```python
from build123d import *

# Parameters (mm, degrees)
SALIENTE_EXTRUIR1_DEPTH = 5
CROQUIS2_R              = 1.563071694
CORTAR_EXTRUIR1_DEPTH   = 10


with BuildPart() as part:
    # Croquis1 → Saliente-Extruir1 (new body)
    with BuildSketch(Plane.XY):
        with BuildLine():
            ThreePointArc((-51.415727165, 73.433311131), (-42.744189857, 73.869405728), (-37.96791411, 81.120124849))
            Line((-37.96791411, 81.120124849), (-37.96791411, 86.394261487))
            Line((-37.96791411, 86.394261487), (-19.296868546, 86.394261487))
            Line((-19.296868546, 86.394261487), (-19.296868546, 91.89912361))
            ThreePointArc((-19.296868546, 91.89912361), (-17.466810584, 93.728616325), (-14.967256479, 94.398231899))
            Line((-14.967256479, 94.398231899), (14.931670067, 94.398231899))
            ThreePointArc((14.931670067, 94.398231899), (17.431224172, 93.728616325), (19.261282134, 91.89912361))
            Line((19.261282134, 91.89912361), (19.261282134, 86.402202311))
            Line((19.261282134, 86.402202311), (49.864249238, 86.408504811))
            Line((49.864249238, 86.408504811), (65.171190916, 59.908709118))
            Line((65.171190916, 59.908709118), (69.938541359, 62.661140179))
            ThreePointArc((69.938541359, 62.661140179), (72.437957507, 61.991009851), (74.267638657, 60.161140285))
            Line((74.267638657, 60.161140285), (89.21710193, 34.267910351))
            ThreePointArc((89.21710193, 34.267910351), (89.886974885, 31.768425211), (89.217616699, 29.268802168))
            Line((89.217616699, 29.268802168), (84.457143211, 26.520341518))
            Line((84.457143211, 26.520341518), (99.764084889, 0.020545825))
            Line((99.764084889, 0.020545825), (84.468059462, -26.485552369))
            Line((84.468059462, -26.485552369), (89.235409905, -29.237983431))
            ThreePointArc((89.235409905, -29.237983431), (89.904768091, -31.737606474), (89.234895136, -34.237091613))
            Line((89.234895136, -34.237091613), (74.285431863, -60.130321548))
            ThreePointArc((74.285431863, -60.130321548), (72.455750713, -61.960191114), (69.956334565, -62.630321442))
            Line((69.956334565, -62.630321442), (65.195861077, -59.881860793))
            Line((65.195861077, -59.881860793), (56.094468632, -75.653435114))
            ThreePointArc((56.094468632, -75.653435114), (42.096374739, -72.88292625), (37.495566471, -86.390513573))
            Line((37.495566471, -86.390513573), (19.296868546, -86.394261487))
            Line((19.296868546, -86.394261487), (19.296868546, -91.89912361))
            ThreePointArc((19.296868546, -91.89912361), (17.466810584, -93.728616325), (14.967256479, -94.398231899))
            Line((14.967256479, -94.398231899), (-14.931670067, -94.398231899))
            ThreePointArc((-14.931670067, -94.398231899), (-17.431224172, -93.728616325), (-19.261282134, -91.89912361))
            Line((-19.261282134, -91.89912361), (-19.261282134, -86.402202311))
            Line((-19.261282134, -86.402202311), (-49.864249238, -86.408504811))
            Line((-49.864249238, -86.408504811), (-65.171190916, -59.908709118))
            Line((-65.171190916, -59.908709118), (-69.938541359, -62.661140179))
            ThreePointArc((-69.938541359, -62.661140179), (-72.437957507, -61.991009851), (-74.267638657, -60.161140285))
            Line((-74.267638657, -60.161140285), (-89.21710193, -34.267910351))
            ThreePointArc((-89.21710193, -34.267910351), (-89.886974885, -31.768425211), (-89.217616699, -29.268802168))
            Line((-89.217616699, -29.268802168), (-84.457143211, -26.520341518))
            Line((-84.457143211, -26.520341518), (-99.764084889, -0.020545825))
            Line((-99.764084889, -0.020545825), (-84.468059462, 26.485552369))
            Line((-84.468059462, 26.485552369), (-89.235409905, 29.237983431))
            ThreePointArc((-89.235409905, 29.237983431), (-89.904768091, 31.737606474), (-89.234895136, 34.237091613))
            Line((-89.234895136, 34.237091613), (-74.285431863, 60.130321548))
            ThreePointArc((-74.285431863, 60.130321548), (-72.455750713, 61.960191114), (-69.956334565, 62.630321442))
            Line((-69.956334565, 62.630321442), (-65.195861077, 59.881860793))
            Line((-65.195861077, 59.881860793), (-55.88668677, 76.013702989))
            Line((-55.88668677, 76.013702989), (-51.415727165, 73.433311131))
        make_face()
    extrude(amount=SALIENTE_EXTRUIR1_DEPTH)

    # Croquis2 → Cortar-Extruir1 (cut)
    with BuildSketch(Plane.XY.offset(5)):
        with Locations((40.934728827, -68.058233997)):
            Circle(CROQUIS2_R)
    extrude(amount=-CORTAR_EXTRUIR1_DEPTH, mode=Mode.SUBTRACT)


solid = part.part
```
The listing builds one solid part. Answer for the finished solid, in the listing's coordinates (mm). A direction names the side the tool comes from. Coordinates: 2 decimals unless noted, no trailing zeros. Loops run counter-clockwise (first coordinate to the right, second up) from the corner with the lowest first, then second, coordinate; pieces in that order, holes last. Notation, with made-up numbers: M 44.5,30.5 L 61.5,30.5 A18 ccw 61.5,36.5 Z; hole C 49.25,-12 d6. An arc over 180 degrees is marked long. Answer as a JSON object with one key per item and string values. Group by question number.
Item 1: Each of these flat-tipped pins is pushed along its axis until it touches: P1, Ø1.5, axis at y = -12.5, z = 2, coming from the +X side; P2, Ø2.5, axis at x = -33, z = 3.5, coming from the +Y side; P3, Ø5, axis at x = 65.5, y = -66.5, coming from the +Z side; P4, Ø1, axis at x = 62, z = 0.5, coming from the -Y side. Where does it stop, or does it pass through?
Item 2: Section B-B (y = 51) is taken. Write down the section's boundary in (x, z), and give its area (3 significant figures).
Item 3: Determine the mould class of faces 1 (the face through (92, 13.46, 2.46)), 2 (the face through (19.297, -89, 2)), 3 (the face through (-72.406, -62.009, 2.465)) for opening direction Y: +Y half, -Y half, draft (parallel to the pull), parting line (faces both ways), or undercut.
Item 4: Section A-A (x = -44.5) is taken. Write down the section's boundary in (y, z).
Item 5: Which of the six approach directions +Z, -Z, +X, -X, +Y, -Y give full straight-line access (tool end or side, diameter ignored) to faces 4 (the face through (0, -94.398, 2)), 5 (the face through (-17.399, -93.747, 2.465)), 6 (the face through (-86.871, -27.914, 2.465)), 7 (the face through (67.521, 61.266, 2.465)), 8 (the face through (86.818, -27.843, 2.465))?
Item 6: Consider L1, parallel to Y at x = 26, z = 0.4; L2, parallel to X at y = -72.5, z = 2.7; L3, parallel to Y at x = -70, z = 2.15. Determine where each line is inside the solid, lowest interval first.
Solved:
{
 "1": {"P1": "stops at x = 92.97", "P2": "stops at y = 86.39", "P3": "passes through", "P4": "stops at y = -66.29"},
 "2": {"outline": "M -79.56,0 L 79.56,0 L 79.56,5 L -79.56,5 Z", "area": "796 mm2"},
 "3": {"face 1": "undercut", "face 2": "draft", "face 3": "-Y half"},
 "4": {"outline": "M -86.41,0 L 73.09,0 L 73.09,5 L -86.41,5 Z"},
 "5": {"face 4": "+Z, -Z, +X, -X, -Y", "face 5": "+Z, -Z, -X, -Y", "face 6": "+Z, -Z, -X", "face 7": "+Z, -Z, +Y", "face 8": "+Z, -Z, +X"},
 "6": {"L1": "y = -86.39 to 86.4", "L2": "x = -57.9 to 42.82, 52.2 to 57.91", "L3": "y = -62.66 to 62.63"}
}
